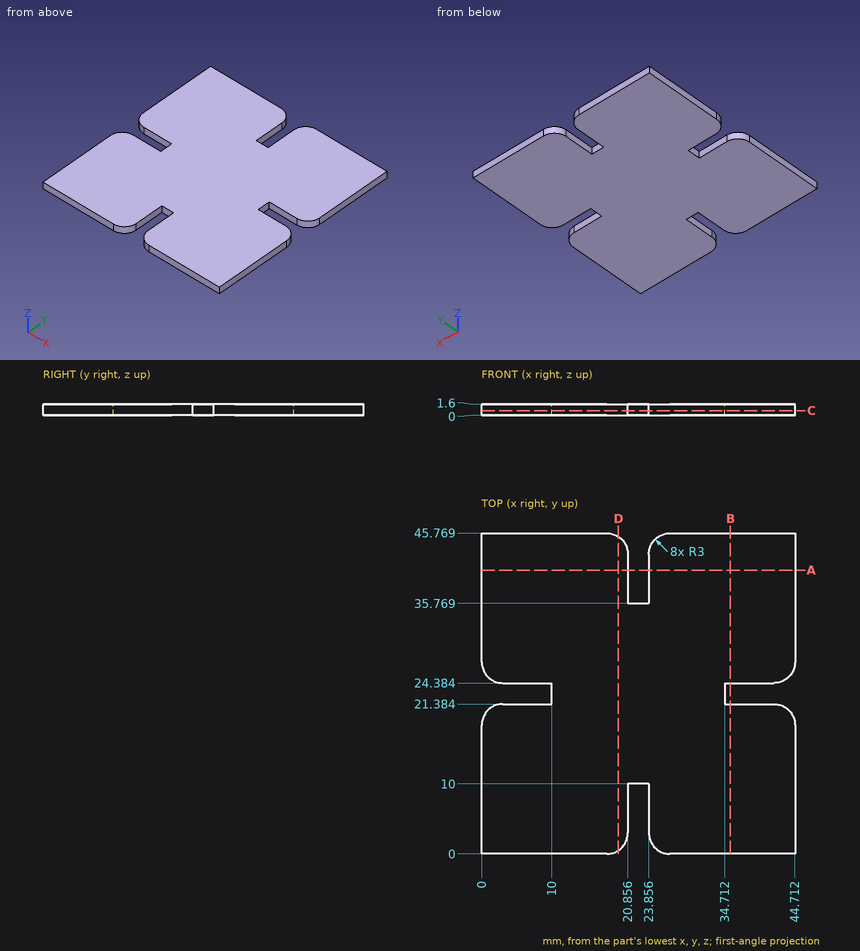
Can you work these out from the drawing? Everything is in mm from the part's minimum corner. Give positions to 0.01 mm unless a question says otherwise; leave off trailing zeros. Write each loop counter-clockwise with the first axis right and the second up, starting at its lowest first coordinate (ties: lowest second). Pieces come first, ordered by that corner, then holes. Notation, with made-up numbers: (-10, -19) -> (33, -19) arc R21 ccw to (33, 9) -> close; hole circle Ø3 at (78, 17). An arc over 180 degrees is marked (long way). Write each question's results on one line, items separated by ' | '.
Item 1: Suppose I cut it at D-D on x = 19.5. Write out the boundary of the cut face in (y, z).
Output:
outline: (0.49, 0) -> (45.28, 0) -> (45.28, 1.6) -> (0.49, 1.6) -> close
Item 2: If I drill on L1, parallel to Y at x = 40.5, z = 0.8 (1 decimal); L2, parallel to X at y = 6, z = 0.65; L3, parallel to Y at x = 18, z = 1.35 (1 decimal), over which ranges is the centre line in solid material (lowest first)?
Output:
L1: y = 0 to 21.4, 24.4 to 45.8 | L2: x = 0 to 20.86, 23.86 to 44.71 | L3: y = 0 to 45.8
Item 3: Suppose I cut it at B-B on x = 35.5. Write out the boundary of the cut face in (y, z) (1 decimal).
Output:
outline: (0, 0) -> (21.4, 0) -> (21.4, 1.6) -> (0, 1.6) -> close; (24.4, 0) -> (45.8, 0) -> (45.8, 1.6) -> (24.4, 1.6) -> close
Item 4: Suppose I cut it at C-C on z = 0.65. Write out the boundary of the cut face in (x, y) (1 decimal), plus the area to 3 significant figures.
Output:
outline: (0, 0) -> (17.9, 0) arc R3 ccw to (20.9, 3) -> (20.9, 10) -> (23.9, 10) -> (23.9, 3) arc R3 ccw to (26.9, 0) -> (44.7, 0) -> (44.7, 18.4) arc R3 ccw to (41.7, 21.4) -> (34.7, 21.4) -> (34.7, 24.4) -> (41.7, 24.4) arc R3 ccw to (44.7, 27.4) -> (44.7, 45.8) -> (26.9, 45.8) arc R3 ccw to (23.9, 42.8) -> (23.9, 35.8) -> (20.9, 35.8) -> (20.9, 42.8) arc R3 ccw to (17.9, 45.8) -> (0, 45.8) -> (0, 27.4) arc R3 ccw to (3, 24.4) -> (10, 24.4) -> (10, 21.4) -> (3, 21.4) arc R3 ccw to (0, 18.4) -> close | area: 1,910 mm^2
Item 5: Suppose I cut it at A-A on y = 40.5. Write out the boundary of the cut face in (x, z).
Output:
outline: (0, 0) -> (20.86, 0) -> (20.86, 1.6) -> (0, 1.6) -> close; (23.86, 0) -> (44.71, 0) -> (44.71, 1.6) -> (23.86, 1.6) -> close
Item 6: For pin 1 Ø12 at (x, y) = (23, 31.5) entering from -Z; pin 2 Ø0.5 at (x, z) = (22, 1) entering from +Y; pin 3 Ø0.5 at (y, z) = (23, 1) entering from +X; pin 4 Ø0.8 at (y, z) = (22.5, 1) entering from -X, each with a flat end and sliding along its axis, tell me the tip position at first contact or that it passes through.
Output:
pin 1: stops at z = 0 | pin 2: stops at y = 35.77 | pin 3: stops at x = 34.71 | pin 4: stops at x = 10
